The listing builds one solid part. Answer for the finished solid, in the listing's coordinates (mm). A direction names the side the tool comes from. Give positions to 0.01 mm unless a question says otherwise; leave off trailing zeros. Loops run counter-clockwise (first coordinate to the right, second up) from the corner with the lowest first, then second, coordinate; pieces in that order, holes last.
Item 1: Section A-A, the plane y = -0.8 is taken. Give the vertices of the cut face in (x, z).
Item 2: Section B-B, the plane z = -8 is taken. Give the vertices of the cut face in (x, y).
Item 3: Consider line 1 along X through (y, z) = (-1.5, -2.75); line 2 along X through (y, z) = (-2.7, 2.25); line 3 along Z through (x, y) = (-109, -4.7). Determine where each line is inside the solid, lowest interval first.
Item 4: Section C-C, the plane z = 3.5 is taken. Give the vertices of the cut face in (x, y), and give its area (3 significant figures).
Item 5: Each of these flat-tipped pins is pushed along its axis until it touches: pin 1 Ø1 at (y, z) = (-1, -2) entering from +X; pin 2 Ø3 at (x, y) = (-167.5, -1.5) entering from +Z; pin 3 Ø2.5 at (x, y) = (-110, -3) entering from -Z; pin 4 Ø5 at (x, z) = (-144.5, -1) entering from +Y. Where does it stop, or does it pass through?
Item 6: Section D-D, the plane x = -128.5 is taken. Give the vertices of the cut face in (y, z), and give its area (3 significant figures).
Item 7: The mould has two halves that part along Z. Classify faces 1 (the face through (-126, -5, 0)), 2 (the face through (-55.086, -2.465, 1.624)), 3 (the face through (-185.086, -2.465, 1.624)), 4 (the face through (-69.614, -2.465, 7.707)): pulls with the +Z half, pulls with the -Z half, needs draft (parallel to the pull), parting line crosses it, or undercut.
Item 8: A tool of negligible diameter and unlimited length cuts with its end or side. For faces 5 (the face through (-179.614, -2.465, -7.293)), 6 (the face through (-126, 0, 0)), 7 (the face through (-125, -2, 5.242)), from which of +Z, -Z, +X, -X, +Y, -Y can it reach the whole face along a straight path? Write none if from no direction.
from build123d import *

# Parameters (mm, degrees)
SKETCH_R     = 4.6
PAD001_DEPTH = 5


with BuildPart() as part:
    # Sketch → Pad001 (new body)
    with BuildSketch(Plane.XZ):
        with BuildLine():
            ThreePointArc((-59.473739, -9.758096), (-49.473739, 0.241904), (-59.473739, 10.241904))
            Line((-79.473739, 5.241904), (-59.473739, 10.241904))
            Line((-169.473739, 5.241904), (-79.473739, 5.241904))
            Line((-189.473739, 10.241904), (-169.473739, 5.241904))
            ThreePointArc((-189.473739, 10.241904), (-199.473739, 0.241904), (-189.473739, -9.758096))
            Line((-189.473739, -9.758096), (-169.473739, -4.758096))
            Line((-169.473739, -4.758096), (-79.473739, -4.758096))
            Line((-79.473739, -4.758096), (-59.473739, -9.758096))
        make_face()
        with Locations((-59.473739, 0.241904)):
            Circle(SKETCH_R, mode=Mode.SUBTRACT)
        with Locations((-189.473739, 0.241904)):
            Circle(SKETCH_R, mode=Mode.SUBTRACT)
    extrude(amount=PAD001_DEPTH)


solid = part.part
Worked answers:
1. outline: (-189.47, -9.76) - (-169.47, -4.76) - (-79.47, -4.76) - (-59.47, -9.76) arc R10 ccw to (-59.47, 10.24) - (-79.47, 5.24) - (-169.47, 5.24) - (-189.47, 10.24) arc R10 ccw to start; hole circle Ø9.2 at (-189.47, 0.24); hole circle Ø9.2 at (-59.47, 0.24)
2. outline: (-195.14, -5) - (-182.44, -5) - (-182.44, 0) - (-195.14, 0) - close; (-66.51, -5) - (-53.81, -5) - (-53.81, 0) - (-66.51, 0) - close
3. line 1: x = -199.02 to -192.97, -185.98 to -62.97, -55.98 to -49.93
3. line 2: x = -199.27 to -193.61, -185.34 to -63.61, -55.34 to -49.68
3. line 3: z = -4.76 to 5.24
4. outline: (-198.93, -5) - (-192.72, -5) - (-192.72, 0) - (-198.93, 0) - close; (-186.23, -5) - (-62.72, -5) - (-62.72, 0) - (-186.23, 0) - close; (-56.23, -5) - (-50.02, -5) - (-50.02, 0) - (-56.23, 0) - close
4. area: 680 mm2
5. pin 1: stops at x = -49.63
5. pin 2: stops at z = 5.24
5. pin 3: stops at z = -4.76
5. pin 4: stops at y = 0
6. outline: (-5, -4.76) - (0, -4.76) - (0, 5.24) - (-5, 5.24) - close
6. area: 50.0 mm2
7. face 1: needs draft
7. face 2: undercut
7. face 3: undercut
7. face 4: pulls with the +Z half
8. face 5: -Z, +Y, -Y
8. face 6: +Z, -Z, +X, -X, +Y
8. face 7: +Z, +Y, -Y
